Model file for the job. Use its own axes, mm. A direction names the side the tool comes from. Give positions to 0.01 mm unless a question says otherwise; leave off trailing zeros. Write each loop counter-clockwise with the first axis right and the second up, starting at its lowest first coordinate (ties: lowest second). Pieces come first, ordered by that corner, then holes. Notation, with made-up numbers: (59, 80) - (97, 80) arc R20 cw to (97, 89) - close; hole circle Ø7 at (12, -35). An arc over 180 degrees is marked (long way). Use CSV: the item, a comma, the result in double quotes.
from build123d import *

# Parameters (mm, degrees)
F1_DEPTH = 9


with BuildPart() as f1:
    # F0 (on Top) → F1 (new body)
    with BuildSketch(Plane.XY):
        with BuildLine():
            Line((-3.572917, 3.353247), (-3.572917, 5.429942))
            ThreePointArc((-3.572917, 5.429942), (-6.215398, 1.90232), (-6, -2.5))
            Line((-6, -2.5), (-6, -5.5))
            Line((-6, -5.5), (-18, -5.5))
            Line((-18, -5.5), (-18, -8.5))
            Line((-18, -8.5), (18, -8.5))
            Line((18, -8.5), (18, -5.5))
            Line((18, -5.5), (6, -5.5))
            Line((6, -5.5), (6, -2.5))
            ThreePointArc((6, -2.5), (6.215398, 1.90232), (3.572917, 5.429942))
            Line((3.572917, 5.429942), (3.572917, 3.353247))
            ThreePointArc((3.572917, 3.353247), (0, -4.9), (-3.572917, 3.353247))
        make_face()
    extrude(amount=F1_DEPTH)


solid = f1.part
(1) Pull direction Y, two halves, no side cores. Call faces 1 (the face through (6.234, 1.842, 4.437)), 2 (the face through (3.573, 4, 4)), 3 (the face through (0, -8.5, 4)): released by +Y, released by -Y, zero draft, split by the parting line, or undercut.
Checked values:
face 1,"undercut"
face 2,"zero draft"
face 3,"released by -Y"
(2) Wall check: probe 1 along X at (y, z) = (0, 2.25); probe 2 along Y at (x, z) = (0, 3); probe 3 along X at (y, z) = (2.75, 8.75). Give the ranges that are in metal, low to high. Write a range as [from, to].
Checked values:
probe 1,"x = [-6.5, -4.9], [4.9, 6.5]"
probe 2,"y = [-8.5, -4.9]"
probe 3,"x = [-5.89, -4.06], [4.06, 5.89]"
(3) Saw through at D-D, the plane x = 0. List the corners of the cut face in (y, z).
Checked values:
outline,"(-8.5, 0) - (-4.9, 0) - (-4.9, 9) - (-8.5, 9) - close"
(4) Saw through at C-C, the plane x = 4. List the corners of the cut face in (y, z), then the cut area to 3 significant figures.
Checked values:
outline,"(-8.5, 0) - (-2.83, 0) - (-2.83, 9) - (-8.5, 9) - close; (2.83, 0) - (5.12, 0) - (5.12, 9) - (2.83, 9) - close"
area,"71.7 mm^2"
(5) Saw through at B-B, the plane z = 4.5. List the corners of the cut face in (x, y), then the cut area to 3 significant figures.
Checked values:
outline,"(-18, -8.5) - (18, -8.5) - (18, -5.5) - (6, -5.5) - (6, -2.5) arc R6.5 ccw to (3.57, 5.43) - (3.57, 3.35) arc R4.9 cw (long way) to (-3.57, 3.35) - (-3.57, 5.43) arc R6.5 ccw to (-6, -2.5) - (-6, -5.5) - (-18, -5.5) - close"
area,"154 mm^2"
(6) 3-axis set-ups, long thin cutter, end or side, ignore diameter. For faces 4 (the face through (-6, -4, 4)), 5 (the face through (-18, -7, 4)), 6 (the face through (6, -4, 4)), 7 (the face through (-3.573, 4, 4)): which of +Z, -Z, +X, -X, +Y, -Y reach the whole face in a straight line?
Checked values:
face 4,"+Z, -Z, -X"
face 5,"+Z, -Z, -X, +Y, -Y"
face 6,"+Z, -Z, +X"
face 7,"+Z, -Z, +Y"
(7) Saw through at A-A, the plane y = 0. List the corners of the cut face in (x, z).
Checked values:
outline,"(-6.5, 0) - (-4.9, 0) - (-4.9, 9) - (-6.5, 9) - close; (4.9, 0) - (6.5, 0) - (6.5, 9) - (4.9, 9) - close"
(8) Flat gauge pins, fed straight in: P1, Ø8, axis at x = 0, y = 0, coming from the +Z side; P2, Ø1, axis at x = -2.5, z = 6.5, coming from the +Y side; P3, Ø2.5, axis at y = 4.5, z = 2.5, coming from the +X side; P4, Ø2.5, axis at y = -4, z = 4.5, coming from the -X side. Where does each tip first touch, or does it go through?
Checked values:
P1,"passes through"
P2,"stops at y = -3.87"
P3,"stops at x = 5.63"
P4,"stops at x = -6"
